from build123d import *

# Parameters (mm, degrees)
ESQUISSE1_W             = 62.2
ESQUISSE1_H             = 10
ESQUISSE1_R             = 1.65
BOSS_EXTRU_1_DEPTH      = 4
BOSS_EXTRU_2_DEPTH      = 3
BOSS_EXTRU_2_DEPTH_BACK = 4
CONG_1_R                = 3
ESQUISSE3_R             = 1.65
BOSS_EXTRU_3_DEPTH      = 7
ENL_V_MAT_EXTRU_1_DEPTH = 2
ESQUISSE6_R             = 3.25
ENL_V_MAT_EXTRU_2_DEPTH = 4
CONG_2_R                = 1


with BuildPart() as part:
    # Esquisse1 → Boss.-Extru.1 (new body)
    with BuildSketch(Plane(origin=(0, 0, 0), x_dir=(1, 0, 0), z_dir=(0, 1, 0))):
        with Locations((0, -1.7)):
            Rectangle(ESQUISSE1_W, ESQUISSE1_H)
        with Locations(Location((-27.8, 0, 0), (0, 0, 270))):
            Circle(ESQUISSE1_R, mode=Mode.SUBTRACT)
        with Locations(Location((27.8, 0, 0), (0, 0, 270))):
            Circle(ESQUISSE1_R, mode=Mode.SUBTRACT)
    extrude(amount=BOSS_EXTRU_1_DEPTH)

    # Esquisse2 → Boss.-Extru.2 (add, two sides: drawn at the far end of the back side and taken through both)
    with BuildSketch(Plane(origin=(0, 4, 0), x_dir=(1, 0, 0), z_dir=(0, 1, 0)).offset(-BOSS_EXTRU_2_DEPTH_BACK)):
        Polygon((-31.1, -6.7), (-31.1, 3.3), (31.1, 3.3), (31.1, -6.7), (33.5, -6.7), (33.5, 5.3), (-33.5, 5.3), (-33.5, -6.7), align=None)
    extrude(amount=BOSS_EXTRU_2_DEPTH + BOSS_EXTRU_2_DEPTH_BACK)

    # Congé1
    cong_1_edges = [part.edges().sort_by_distance(p)[0] for p in [
        (31.1, 5.5, -3.3),
        (-31.1, 5.5, -3.3),
    ]]
    fillet(cong_1_edges, radius=CONG_1_R)

    # Esquisse3 → Boss.-Extru.3 (add)
    # profile 1 of 2: a face of its own
    with BuildSketch(Plane(origin=(0, 7, 0), x_dir=(1, 0, 0), z_dir=(0, 1, 0))):
        with BuildLine():
            Line((-39, 5.3), (-33.5, 5.3))
            Line((-33.5, 5.3), (-33.5, -6.7))
            Line((-33.5, -6.7), (-39, -6.7))
            ThreePointArc((-39, -6.7), (-45, -0.7), (-39, 5.3))
        make_face()
        with Locations(Location((-36.5, -0.7, 0), (0, 0, 270))):
            Circle(ESQUISSE3_R, mode=Mode.SUBTRACT)
    # profile 2 of 2: a face of its own
    with BuildSketch(Plane(origin=(0, 7, 0), x_dir=(1, 0, 0), z_dir=(0, 1, 0))):
        with BuildLine():
            Line((33.5, 5.3), (33.5, -6.7))
            Line((33.5, -6.7), (39, -6.7))
            ThreePointArc((39, -6.7), (45, -0.7), (39, 5.3))
            Line((39, 5.3), (33.5, 5.3))
        make_face()
        with Locations(Location((36.5, -0.7, 0), (0, 0, 90))):
            Circle(ESQUISSE3_R, mode=Mode.SUBTRACT)
    extrude(amount=-BOSS_EXTRU_3_DEPTH)

    # Esquisse5 → Enlèv. mat.-Extru.1 (cut)
    with BuildSketch(Plane.XZ):
        Polygon((-29.445448267, 2.85), (-26.154551733, 2.85), (-24.509103466, 0), (-26.154551733, -2.85), (-29.445448267, -2.85), (-31.090896534, 0), align=None)
        Polygon((26.154551733, 2.85), (29.445448267, 2.85), (31.090896534, 0), (29.445448267, -2.85), (26.154551733, -2.85), (24.509103466, 0), align=None)
    extrude(amount=-ENL_V_MAT_EXTRU_1_DEPTH, mode=Mode.SUBTRACT)

    # Esquisse6 → Enlèv. mat.-Extru.2 (cut)
    with BuildSketch(Plane(origin=(0, 7, 0), x_dir=(1, 0, 0), z_dir=(0, 1, 0))):
        with Locations(Location((-36.5, -0.7, 0), (0, 0, 270))):
            Circle(ESQUISSE6_R)
        with Locations(Location((36.5, -0.7, 0), (0, 0, 270))):
            Circle(ESQUISSE6_R)
    extrude(amount=-ENL_V_MAT_EXTRU_2_DEPTH, mode=Mode.SUBTRACT)

    # Congé2
    cong_2_edges = [part.edges().sort_by_distance(p)[0] for p in [
        (0, 4, 6.7),
        (31.1, 5.5, 6.7),
        (0, 0, -5.3),
        (-31.1, 5.5, 6.7),
        (-35.05, 7, 6.7),
        (-31.1, 7, 3.2),
        (35.05, 7, 6.7),
        (0, 7, -5.3),
        (0, 7, -3.3),
        (31.1, 7, 3.2),
        (0, 0, 6.7),
        (30.221320344, 7, -2.421320344),
        (-30.221320344, 7, -2.421320344),
        (-45, 0, 0.7),
        (-45, 7, 0.7),
        (45, 0, 0.7),
        (45, 7, 0.7),
    ]]
    fillet(cong_2_edges, radius=CONG_2_R - 0.0001)  # a hair under: the kernel refuses the full size


solid = part.part
Read the model definition and answer for the solid it produces. Units are mm, in the model's axes. A direction names the side the tool comes from. Round coordinates to 2 decimals unless told otherwise and drop trailing zeros. Loops run counter-clockwise (first coordinate to the right, second up) from the corner with the lowest first, then second, coordinate; pieces in that order, holes last.
Q1. Section B-B on y = 5 is taken. Write down the section's boundary in (x, z), and give its area (3 significant figures).
Q2. Section A-A on x = 36.5 is taken. Write down the section's boundary in (y, z), and give its area (3 significant figures).
Q3. Consider probe 1 along X at (y, z) = (4.6, 0.7); probe 2 along Z at (x, y) = (36.5, 1.7); probe 3 along X at (y, z) = (2.75, 0.75). Determine where each line is inside the solid, lowest interval first.
Q4. Each of these flat-tipped pins is pushed along its axis until it touches: pin 1 (5.5 mm diameter, centred on x = 27.8, z = 0, fed in from -Y); pin 2 (6 mm diameter, centred on x = -11, z = 1.5, fed in from +Y); pin 3 (0.6 mm diameter, centred on y = 4.5, z = 2, fed in from -X). Where does it stop, or does it pass through?
Q5. Which of the six approach directions +Z, -Z, +X, -X, +Y, -Y give full straight-line access (tool end or side, diameter ignored) to faces 4 (the face through (-31.1, 5, 3)), 5 (the face through (35, 3, 2)), 6 (the face through (1, 0, 1)), 7 (the face through (30.28, 0.986, -1.405))?
Q6. Determine the mould class of faces 1 (the face through (25.32, 0.986, 1.405)), 2 (the face through (-1, 4, -5.3)), 3 (the face through (-30.24, 5.01, -2.4)) for opening direction Z: released by +Z, released by -Z, zero draft, split by the parting line, or undercut.
Output:
1. outline: (-39, -5.3) - (39, -5.3) arc R6 ccw to (39, 6.7) - (32.1, 6.7) arc R1 ccw to (31.1, 5.7) - (31.1, -0.3) arc R3 cw to (28.1, -3.3) - (-28.1, -3.3) arc R3 cw to (-31.1, -0.3) - (-31.1, 5.7) arc R1 ccw to (-32.1, 6.7) - (-39, 6.7) arc R6 ccw to start; hole circle Ø6.5 at (-36.5, 0.7); hole circle Ø6.5 at (36.5, 0.7)
1. area: 364 mm2
2. outline: (0, -4.3) arc R1 ccw to (1, -5.3) - (6, -5.3) arc R1 ccw to (7, -4.3) - (7, -2.55) - (3, -2.55) - (3, -0.95) - (0, -0.95) - close; (0, 2.35) - (3, 2.35) - (3, 3.95) - (7, 3.95) - (7, 5.7) arc R1 ccw to (6, 6.7) - (1, 6.7) arc R1 ccw to (0, 5.7) - close
2. area: 47.2 mm2
3. probe 1: x = -45 to -39.75, -33.25 to -31.1, 31.1 to 33.25, 39.75 to 45
3. probe 2: z = -5.3 to -0.95, 2.35 to 6.7
3. probe 3: x = -45 to -38.15, -34.85 to -29.27, -26.33 to 26.33, 29.27 to 34.85, 38.15 to 45
4. pin 1: stops at y = 2
4. pin 2: stops at y = 4
4. pin 3: stops at x = -44.92
5. face 4: +Z, +Y
5. face 5: +Y
5. face 6: +Z, -Z, +X, -X, -Y
5. face 7: -Y
6. face 1: undercut
6. face 2: released by -Z
6. face 3: released by +Z
